```python
from build123d import *

# Parameters (mm, degrees)
SKETCH_1_W           = 70
SKETCH_1_H           = 40
EXTRUDE_1_DEPTH      = 30
EXTRUDE_3_DEPTH      = 200
EXTRUDE_3_DEPTH_BACK = 35
SKETCH_5_W           = 70
SKETCH_5_H           = 2.954129794
SKETCH_6_W           = 70
SKETCH_6_H           = 6
EXTRUDE_4_DEPTH      = 40
SKETCH_8_R           = 1.75
CUT_EXTRUDE_1_DEPTH  = 6
SKETCH_9_R           = 4
CUT_EXTRUDE_2_DEPTH  = 6


with BuildPart() as part:
    # 草图1 → 凸台-拉伸1 (new body)
    with BuildSketch(Plane(origin=(0, 0, 0), x_dir=(1, 0, 0), z_dir=(0, 1, 0))):
        with Locations((35, 20)):
            Rectangle(SKETCH_1_W, SKETCH_1_H)
    extrude(amount=EXTRUDE_1_DEPTH)

    # 草图5 → 凸台-拉伸3 (add, two sides: drawn at the far end of the back side and taken through both)
    with BuildSketch(Plane(origin=(0, 0, 0), x_dir=(1, 0, 0), z_dir=(0, 1, 0)).offset(-EXTRUDE_3_DEPTH_BACK)):
        with Locations((35, -1.477064897)):
            Rectangle(SKETCH_5_W, SKETCH_5_H)
    extrude(amount=EXTRUDE_3_DEPTH + EXTRUDE_3_DEPTH_BACK)

    # 草图6 → 凸台-拉伸4 (add)
    with BuildSketch(Plane.XY.offset(2.954129794)):
        with Locations((35, -32)):
            Rectangle(SKETCH_6_W, SKETCH_6_H)
    extrude_4 = extrude(amount=EXTRUDE_4_DEPTH)

    # 镜向1: 凸台-拉伸4 across plane
    add(extrude_4.mirror(Plane.ZX.offset(82.5)))

    # 草图8 → 切除-拉伸1 (cut)
    with BuildSketch(Plane.XZ):
        with Locations(Location((60, -5, 0), (0, 0, 270))):
            Circle(SKETCH_8_R)
        with Locations(Location((10, -5, 0), (0, 0, 90))):
            Circle(SKETCH_8_R)
        with Locations(Location((60, -30, 0), (0, 0, 270))):
            Circle(SKETCH_8_R)
        with Locations(Location((10, -30, 0), (0, 0, 90))):
            Circle(SKETCH_8_R)
    extrude(amount=-CUT_EXTRUDE_1_DEPTH, mode=Mode.SUBTRACT)

    # 草图9 → 切除-拉伸2 (cut)
    with BuildSketch(Plane(origin=(0, 200, 0), x_dir=(1, 0, 0), z_dir=(0, 1, 0))):
        with Locations(Location((35, -21.477064897, 0), (0, 0, 270))):
            Circle(SKETCH_9_R)
        with Locations(Location((60, -21.477064897, 0), (0, 0, 270))):
            Circle(SKETCH_9_R)
        with Locations(Location((10, -21.477064897, 0), (0, 0, 90))):
            Circle(SKETCH_9_R)
    cut_extrude_2 = extrude(amount=-CUT_EXTRUDE_2_DEPTH, mode=Mode.SUBTRACT)

    # 镜向2: 切除-拉伸2 across plane
    add(cut_extrude_2.mirror(Plane.ZX.offset(82.5)), mode=Mode.SUBTRACT)


solid = part.part
```
Source: CAD feature listing. Evaluate the final solid. Frame: model axes, mm. A direction names the side the tool comes from. Round coordinates to 2 decimals unless told otherwise and drop trailing zeros. Loops run counter-clockwise (first coordinate to the right, second up) from the corner with the lowest first, then second, coordinate; pieces in that order, holes last. Notation, with made-up numbers: M -9.5,68.5 L 0.5,68.5 A22 cw 0.5,79.5 Z; hole C 44.5,65 d1. An arc over 180 degrees is marked long. Use a Markdown table: item, result. Add a question column.
1. Cut plane B-B, the plane x = 35. Output: boundary loops of the cut face in (y, z), and give its area (3 significant figures).
2. Pull-direction query (Z, two-part tool) for faces 1 (the flat face through (35, 81, 2.954)), 2 (the flat face through (0, 57, 1)), 3 (the cylindrical face through (38.37, -32.04, 23.63)); classes: +Z half, -Z half, draft (parallel to the pull), parting line (faces both ways), or undercut.
3. Cut plane A-A, the plane z = 13. Output: boundary loops of the cut face in (x, y), and give its area (3 significant figures).
4. Cut plane D-D, the plane z = -23.5. Output: boundary loops of the cut face in (x, y).
5. Contact query for flat-ended pins moving along their axis: pin 1 (12 mm diameter, centred on x = 13.5, y = 78.5, fed in from -Z); pin 2 (5.5 mm diameter, centred on x = 60, z = -30, fed in from -Y); pin 3 (21 mm diameter, centred on x = 50.5, y = 52, fed in from +Z). Output: stop coordinate, or through.
6. Ray query, line 1 along X through (y, z) = (2.05, -5); line 2 along Y through (x, z) = (41.5, 32); line 3 along Z through (x, y) = (10, -33). Return the intervals inside material, ascending. Write a range as [from, to].
7. Cut plane C-C, the plane y = 55. Output: boundary loops of the cut face in (x, z).
8. Set-up query: faces 4 (the flat face through (35, 194, 27)), 5 (the flat face through (35, 30, -20)), 6 (the flat face through (35, 0, -20)). Return all of +Z, -Z, +X, -X, +Y, -Y with unobstructed straight access to the full face (end or side cutting, diameter ignored); none if empty.
Solution:
| question | item | result |
|---|---|---|
| 1 | outline | M -35,0 L 0,0 L 0,-40 L 30,-40 L 30,0 L 200,0 L 200,17.48 L 194,17.48 L 194,2.95 L -29,2.95 L -29,17.48 L -35,17.48 Z; M -35,25.48 L -29,25.48 L -29,42.95 L -35,42.95 Z; M 194,25.48 L 200,25.48 L 200,42.95 L 194,42.95 Z |
| 1 | area | 2,280 mm2 |
| 2 | face 1 | +Z half |
| 2 | face 2 | draft |
| 2 | face 3 | undercut |
| 3 | outline | M 0,-35 L 70,-35 L 70,-29 L 0,-29 Z; M 0,194 L 70,194 L 70,200 L 0,200 Z |
| 3 | area | 840 mm2 |
| 4 | outline | M 0,0 L 70,0 L 70,30 L 0,30 Z |
| 5 | pin 1 | stops at z = 0 |
| 5 | pin 2 | stops at y = 0 |
| 5 | pin 3 | stops at z = 2.95 |
| 6 | line 1 | x = [0, 8.25], [11.75, 58.25], [61.75, 70] |
| 6 | line 2 | y = [-35, -29], [194, 200] |
| 6 | line 3 | z = [0, 17.48], [25.48, 42.95] |
| 7 | outline | M 0,0 L 70,0 L 70,2.95 L 0,2.95 Z |
| 8 | face 4 | +Z, +X, -X |
| 8 | face 5 | -Z, +X, -X, +Y |
| 8 | face 6 | -Z, +X, -X, -Y |
